Could you check a few things on this model? Use its own coordinates, in mm. Give positions to 0.01 mm unless a question says otherwise; leave off trailing zeros. Write each loop counter-clockwise with the first axis right and the second up, starting at its lowest first coordinate (ties: lowest second). Pieces come first, ordered by that corner, then holes. Notation, with made-up numbers: (43.5, 64) - (101.5, 64) arc R27 ccw to (101.5, 98) - close; hole circle Ø7 at (34.5, 25). An arc over 180 degrees is marked (long way). Answer as CSV lines item,"result". Start each with the question number.
Q1. Imagine slicing it at D-D on x = 15. List the corners of the cut face in (y, z) for me.
Q2. Will this pin go through, and if not, where does the flat tip stop? pin 1 Ø6 at (x, z) = (43, -69) entering from -Y.
Q3. Imagine slicing it at C-C on y = 0.95. List the corners of the cut face in (x, z) for me, and give its area (3 significant figures).
Q4. If I drill on line 1 along X through (y, z) = (1.7, -15); line 2 along Z through (x, y) = (77.5, 3.55); line 3 along X through (y, z) = (3.75, -75), over which ranges is the centre line in solid material (lowest first)?
Q5. Imagine slicing it at A-A on z = -75. List the corners of the cut face in (x, y) for me.
Q6. Imagine slicing it at B-B on x = 75. List the corners of the cut face in (y, z) for me, and give its area (3 significant figures).
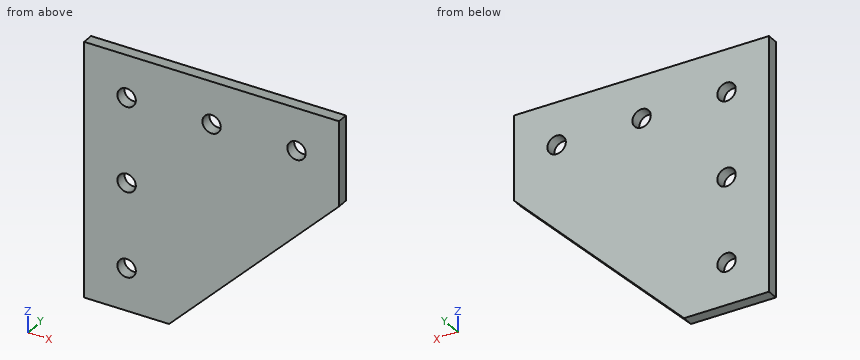
```python
from build123d import *

# Parameters (mm, degrees)
BOSS_EXTRUDE1_DEPTH = 4
SKETCH2_R           = 3.25
CUT_EXTRUDE1_DEPTH  = 128.342059038


with BuildPart() as part:
    # Sketch1 → Boss-Extrude1 (new body)
    with BuildSketch(Plane(origin=(0, 0, 0), x_dir=(1, 0, 0), z_dir=(0, 1, 0))):
        Polygon((0, 0), (90, 0), (90, 30), (30, 90), (0, 90), align=None)
    extrude(amount=BOSS_EXTRUDE1_DEPTH)

    # Sketch2 → Cut-Extrude1 (cut, through all)
    with BuildSketch(Plane(origin=(0, 4, 0), x_dir=(1, 0, 0), z_dir=(0, 1, 0))):
        with Locations(Location((15, 15, 0), (0, 0, 270))):
            Circle(SKETCH2_R)
        with Locations(Location((45, 15, 0), (0, 0, 270))):
            Circle(SKETCH2_R)
        with Locations(Location((75, 15, 0), (0, 0, 270))):
            Circle(SKETCH2_R)
        with Locations(Location((15, 45, 0), (0, 0, 270))):
            Circle(SKETCH2_R)
        with Locations(Location((15, 75, 0), (0, 0, 270))):
            Circle(SKETCH2_R)
    extrude(amount=-CUT_EXTRUDE1_DEPTH, mode=Mode.SUBTRACT)


solid = part.part
```
Conclusion:
1,outline,"(0, -90) - (4, -90) - (4, -78.25) - (0, -78.25) - close; (0, -71.75) - (4, -71.75) - (4, -48.25) - (0, -48.25) - close; (0, -41.75) - (4, -41.75) - (4, -18.25) - (0, -18.25) - close; (0, -11.75) - (4, -11.75) - (4, 0) - (0, 0) - close"
2,pin 1,"y = 0"
3,outline,"(0, -90) - (30, -90) - (90, -30) - (90, 0) - (0, 0) - close; hole circle Ø6.5 at (15, -75); hole circle Ø6.5 at (15, -45); hole circle Ø6.5 at (15, -15); hole circle Ø6.5 at (45, -15); hole circle Ø6.5 at (75, -15)"
3,area,"6,130 mm^2"
4,line 1,"0 to 11.75, 18.25 to 41.75, 48.25 to 71.75, 78.25 to 90"
4,line 2,"-42.5 to -17.08, -12.92 to 0"
4,line 3,"0 to 11.75, 18.25 to 45"
5,outline,"(0, 0) - (11.75, 0) - (11.75, 4) - (0, 4) - close; (18.25, 0) - (45, 0) - (45, 4) - (18.25, 4) - close"
6,outline,"(0, -45) - (4, -45) - (4, -18.25) - (0, -18.25) - close; (0, -11.75) - (4, -11.75) - (4, 0) - (0, 0) - close"
6,area,"154 mm^2"
